Part print with two shaded views. Sizes in mm from the minimum x, y, z corner. A direction names the side the tool comes from. Round coordinates to 2 decimals unless told otherwise and drop trailing zeros. Write each loop counter-clockwise with the first axis right and the second up, starting at its lowest first coordinate (ties: lowest second). Pieces come first, ordered by that corner, then holes.
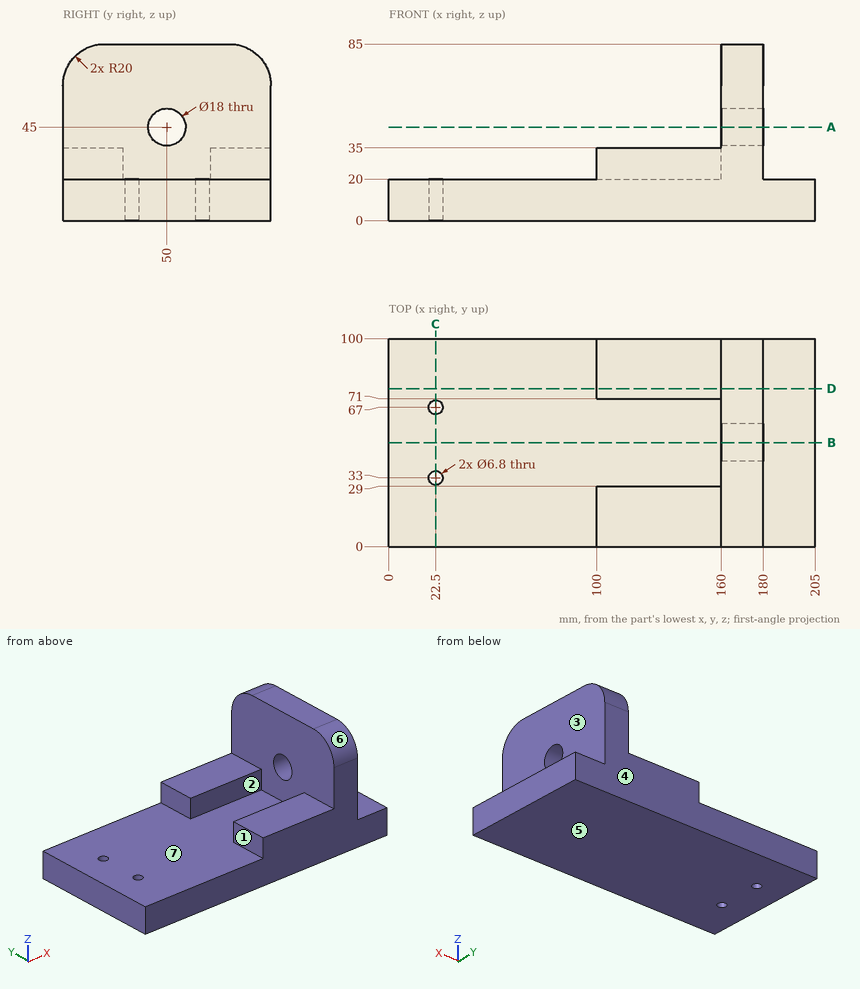
Q1. Wall check: L1, parallel to Y at x = 22.5, z = 6; L2, parallel to Y at x = 165, z = 45; L3, parallel to Z at x = 70, y = 28.5. Give the ranges that are in metal, low to high.
Values follow:
L1: y = 0 to 29.6, 36.4 to 63.6, 70.4 to 100
L2: y = 0 to 41, 59 to 100
L3: z = 0 to 20
Q2. Cut at A-A on z = 45. Write the cut outline in (x, y), plus the area to 3 significant figures.
Values follow:
outline: (160, 0) - (180, 0) - (180, 41) - (160, 41) - close; (160, 59) - (180, 59) - (180, 100) - (160, 100) - close
area: 1,640 mm2
Q3. Cut at D-D on y = 76. Write the cut outline in (x, z), plus the area to 3 significant figures.
Values follow:
outline: (0, 0) - (205, 0) - (205, 20) - (180, 20) - (180, 85) - (160, 85) - (160, 35) - (100, 35) - (100, 20) - (0, 20) - close
area: 6,300 mm2
Q4. Drop flat-ended pins along their axis: pin 1 (1 mm diameter, centred on y = 33, z = 35, fed in from -X); pin 2 (4.5 mm diameter, centred on y = 17, z = 25.5, fed in from -X); pin 3 (14.5 mm diameter, centred on x = 139.5, y = 16.5, fed in from +Z). Give the stop position or say it passes through.
Values follow:
pin 1: stops at x = 160
pin 2: stops at x = 100
pin 3: stops at z = 35
Q5. Cut at C-C on x = 22.5. Write the cut outline in (y, z), plus the area to 3 significant figures.
Values follow:
outline: (0, 0) - (29.6, 0) - (29.6, 20) - (0, 20) - close; (36.4, 0) - (63.6, 0) - (63.6, 20) - (36.4, 20) - close; (70.4, 0) - (100, 0) - (100, 20) - (70.4, 20) - close
area: 1,730 mm2
Q6. Mould opens along Y. For the marked faces 5, 6 and 7 say: +Y half, -Y half, draft (parallel to the pull), parting line (faces both ways), or undercut.
Values follow:
face 5: draft
face 6: -Y half
face 7: undercut
Q7. Which spindle directions (+Z, -Z, +X, -X, +Y, -Y) get a long thin tool onto all of the face, cutting with end or side? Do the marked faces 1, 2, 3 and 4. Say none if no direction does.
Values follow:
face 1: +Z, -X, +Y, -Y
face 2: +Z, -X
face 3: +Z, +X, +Y, -Y
face 4: +Z, -Z, +X, -X, +Y
Q8. Cut at B-B on y = 50. Write the cut outline in (x, z).
Values follow:
outline: (0, 0) - (205, 0) - (205, 20) - (180, 20) - (180, 36) - (160, 36) - (160, 20) - (0, 20) - close; (160, 54) - (180, 54) - (180, 85) - (160, 85) - close
